Verification items for the finished model (mm, model axes). A direction names the side the tool comes from. Coordinates: 2 decimals unless noted, no trailing zeros. Order: outer loops, then holes, each group sorted by start corner. A loop starts at its lowest first (then second) coordinate and runs counter-clockwise, first axis right, second up. Notation, with made-up numbers: M 34,-21.5 L 38,-21.5 A31 ccw 38,4.5 Z; hole C 17,40.25 d6. An arc over 180 degrees is marked long. Return JSON: item names as keys, results as strings. Group by question number.
1. Material ranges on line 1 along Y through (x, z) = (-21.5, 0.9); line 2 along X through (y, z) = (18, 0.2); line 3 along Y through (x, z) = (0, 0.8), recorded low to high.
2. Section check B-B, the plane y = 15.5. Record the cut outline in (x, z), plus the area to 3 significant figures.
3. Section check D-D, the plane z = 1.25. Give the number of separate pieces and of enclosed holes in the cut face, plus the area to 3 significant figures.
4. Gauge pin test, flat ends, axial feed: pin 1 (12 mm diameter, centred on x = -15, y = 5, fed in from +Z); pin 2 (0.8 mm diameter, centred on y = -10.5, z = 0.5, fed in from +X). Record the tip position at first contact, or that the pin passes through.
5. Section check A-A, the plane x = -23.46. Record the cut outline in (y, z).
6. Set-up check for faces 4 (the cylindrical face through (-27.78, 10.25, 0.76)), 5 (the flat face through (2, -12, 1)), 6 (the cylindrical face through (2.179, 7.967, 0.76)): record each of +Z, -Z, +X, -X, +Y, -Y from which the full face is reachable in a straight line by a thin tool's end or side.
7. Section check C-C, the plane x = 5.5. Record the cut outline in (y, z), plus the area to 3 significant figures.
8. Mould release check, pull along X, two halves, no side actions. Record for faces 1 (the flat face through (2, 17, 1)), 2 (the flat face through (-31, 6, 1)), 3 (the flat face through (-4.49, 23, 1)): +X half, -X half, draft (parallel to the pull), parting line (faces both ways), or undercut.
Autodesk Inventor part; units mm, degrees
ref_plane "YZ Plane" through (0, 0, 0) normal (1, 0, 0) x (0, 1, 0)
ref_plane "XZ Plane" through (0, 0, 0) normal (0, 1, 0) x (-1, 0, 0)
ref_plane "XY Plane" through (0, 0, 0) normal (0, 0, 1) x (1, 0, 0)
sketch "スケッチ1" plane through (0, 0, 0) normal (0, 0, 1) x (1, 0, 0)
  circle A0 centre (0, 0) radius 6.05
  arc A1 (2, -7.7976) -> (2, 7.7976) centre (0, 0) ccw
  line L0 (-31, 0) -> (0, 0) construction
  line L1 (-24.51, 24.01) -> (-4.49, 24.01)
  line L2 (-4.49, 24.01) -> (-4.49, 21.99)
  line L3 (-4.49, 21.99) -> (-24.51, 21.99)
  line L4 (-24.51, 21.99) -> (-24.51, 24.01)
  line L5 (-24.51, 24.01) -> (-4.49, 21.99) construction
  line L6 (-4.49, 24.01) -> (-24.51, 21.99) construction
  line L7 (-24.5, 24) -> (-4.5, 24) construction
  line L8 (-4.5, 24) -> (-4.5, 22) construction
  line L9 (-4.5, 22) -> (-24.5, 22) construction
  line L10 (-24.5, 22) -> (-24.5, 24) construction
  line L11 (-24.5, 24) -> (-4.5, 22) construction
  line L12 (-4.5, 24) -> (-24.5, 22) construction
  line L13 (-24.51, 23) -> (-4.49, 23) construction
  arc A2 (-22.41, 24.01) -> (-24.51, 24.01) centre (-23.46, 24.01) ccw
  arc A3 (-24.51, 21.99) -> (-22.41, 21.99) centre (-23.46, 21.99) ccw
  line L14 (-14.5, 24) -> (-14.5, 21.99) construction
  arc A4 (-4.49, 24.01) -> (-6.59, 24.01) centre (-5.54, 24.01) ccw
  arc A5 (-6.59, 21.99) -> (-4.49, 21.99) centre (-5.54, 21.99) ccw
  line L15 (-28, 13.5) -> (-1, 13.5) construction
  line L16 (-1, 13.5) -> (-1, -13.5) construction
  line L17 (-1, -13.5) -> (-28, -13.5) construction
  line L18 (-28, -13.5) -> (-28, 13.5) construction
  line L19 (-28, 13.5) -> (-1, -13.5) construction
  line L20 (-1, 13.5) -> (-28, -13.5) construction
  line L21 (-14.5, 13.5) -> (-14.5, -13.5) construction
  line L22 (-24.51, -10.49) -> (-4.49, -10.49)
  line L23 (-4.49, -10.49) -> (-4.49, -12.51)
  line L24 (-4.49, -12.51) -> (-24.51, -12.51)
  line L25 (-24.51, -12.51) -> (-24.51, -10.49)
  line L26 (-24.51, -10.49) -> (-4.49, -12.51) construction
  line L27 (-4.49, -10.49) -> (-24.51, -12.51) construction
  line L28 (-24.5, -10.5) -> (-4.5, -10.5) construction
  line L29 (-4.5, -10.5) -> (-4.5, -12.5) construction
  line L30 (-4.5, -12.5) -> (-24.5, -12.5) construction
  line L31 (-24.5, -12.5) -> (-24.5, -10.5) construction
  line L32 (-24.5, -10.5) -> (-4.5, -12.5) construction
  line L33 (-4.5, -10.5) -> (-24.5, -12.5) construction
  line L34 (-24.51, -11.5) -> (-4.49, -11.5) construction
  arc A6 (-22.41, -10.49) -> (-24.51, -10.49) centre (-23.46, -10.49) ccw
  arc A7 (-24.51, -12.51) -> (-22.41, -12.51) centre (-23.46, -12.51) ccw
  line L35 (-14.5, -10.5) -> (-14.5, -12.51) construction
  arc A8 (-4.49, -10.49) -> (-6.59, -10.49) centre (-5.54, -10.49) ccw
  arc A9 (-6.59, -12.51) -> (-4.49, -12.51) centre (-5.54, -12.51) ccw
  line L36 (-31, 27) -> (-31, -16.5)
  line L37 (-31, -16.5) -> (2, -16.5)
  line L38 (2, -16.5) -> (2, -7.7976)
  line L39 (2, 7.7976) -> (2, 27)
  line L40 (2, 27) -> (-31, 27)
  arc A10 (-28, 10.5) -> (-25, 13.5) centre (-28, 13.5) ccw
  line L41 (-28, 10.5) -> (-28, 10.5)
  line L42 (-28, 10.5) -> (-28, -7.5)
  line L43 (-28, -7.5) -> (-8.05, -7.5)
  line L44 (-8.05, -7.5) -> (-8.05, 0)
  line L45 (-25, 13.5) -> (-25, 19)
  line L46 (-25, 19) -> (-4, 19)
  arc A11 (-1, 7.9876) -> (-8.05, 0) centre (0, 0) ccw
  line L47 (-1, 9.5) -> (-1, 7.9876)
  circle A12 centre (-28, 13.5) radius 1.35
  arc A13 (0.35, 13.5) -> (-2.35, 13.5) centre (-1, 13.5) ccw
  arc A14 (-2.35, 12.5) -> (0.35, 12.5) centre (-1, 12.5) ccw
  arc A15 (-4, 12.5) -> (-1, 9.5) centre (-1, 12.5) ccw
  line L48 (0.35, 12.5) -> (0.35, 13.5)
  line L49 (-2.35, 13.5) -> (-2.35, 12.5)
  line L50 (-4, 19) -> (-4, 12.5)
  arc A16 (-2.35, -13.5) -> (0.35, -13.5) centre (-1, -13.5) ccw
  arc A17 (0.35, -12.5) -> (-2.35, -12.5) centre (-1, -12.5) ccw
  line L51 (0.35, -12.5) -> (0.35, -13.5)
  line L52 (-2.35, -13.5) -> (-2.35, -12.5)
  circle A18 centre (-28, -13.5) radius 1.35
  point P0 (-14.5, 23)
  point P1 (-14.5, 0)
  point P2 (-14.5, -11.5)
  point P3 (-14.5, 22.995)
  point P4 (-6.59, -10.49)
  point P5 (-6.59, -12.51)
  point P6 (-22.41, -12.51)
  point P7 (-6.59, 24.01)
  dimension "d96" = 12.1
  dimension "d215" = 20
  dimension "d216" = 2
  dimension "d217" = 0.01
  dimension "d219" = 0.01
  dimension "d220" = 1.05
  dimension "d222" = 27
  dimension "d223" = 27
  dimension "d226" = 20
  dimension "d227" = 2
  dimension "d228" = 0.01
  dimension "d229" = 0.01
  dimension "d230" = 1.05
  dimension "d231" = 32.5
  dimension "d238" = 3
  dimension "d240" = 3
  dimension "d241" = 3
  dimension "d242" = 4
  dimension "d243" = 3
  dimension "d244" = 2
  dimension "d245" = 3
  dimension "d246" = 3
  dimension "d247" = 3
  dimension "d248" = 3
  dimension "d251" = 2
  dimension "d252" = 3
  dimension "d255" = 1
  dimension "d257" = 2.7
  dimension "d259" = 2.7
  dimension "d260" = 1
  dimension "d262" = 3
extrude "押し出し1" add sketch "スケッチ1" along normal blind 1.5
fillet "フィレット1" radius 1 7 edges at (-1, 7.9876, 0.75) (-8.05, -7.5, 0.75) (-28, -7.5, 0.75) (-25, 19, 0.75) (-28, 10.5, 0.75) (-4, 19, 0.75) (-1, 9.5, 0.75)
fillet "フィレット2" radius 1 6 edges at (-31, 27, 0.75) (2, 27, 0.75) (-31, -16.5, 0.75) (2, -7.7976, 0.75) (2, -16.5, 0.75) (2, 7.7976, 0.75)
properties part number "Trunk_vertical_frame_06" material "アルミニウム 2014-T4"
Answers follow:
{
 "1": {"line 1": "-16.5 to -12.51, -10.49 to -7.5, 19 to 21.99, 24.01 to 27", "line 2": "-31 to -25, -4 to 2", "line 3": "-16.5 to -14.41, -11.59 to -6.05, 6.05 to 11.59, 14.41 to 27"},
 "2": {"outline": "M -31,0 L -25,0 L -25,1.5 L -31,1.5 Z; M -4,0 L 2,0 L 2,1.5 L -4,1.5 Z", "area": "18.0 mm^2"},
 "3": {"separate pieces": "1", "enclosed holes": "8", "area": "699 mm^2"},
 "4": {"pin 1": "through", "pin 2": "x = 2"},
 "5": {"outline": "M -16.5,0 L -13.56,0 L -13.56,1.5 L -16.5,1.5 Z; M -9.44,0 L -7.5,0 L -7.5,1.5 L -9.44,1.5 Z; M 19,0 L 20.94,0 L 20.94,1.5 L 19,1.5 Z; M 25.06,0 L 27,0 L 27,1.5 L 25.06,1.5 Z"},
 "6": {"face 4": "+Z, -Z", "face 5": "+Z, -Z, +X, -Y", "face 6": "+Z, -Z, +X, +Y"},
 "7": {"outline": "M -5.88,0 L -2.52,0 L -2.52,1.5 L -5.88,1.5 Z; M 2.52,0 L 5.88,0 L 5.88,1.5 L 2.52,1.5 Z", "area": "10.1 mm^2"},
 "8": {"face 1": "+X half", "face 2": "-X half", "face 3": "undercut"}
}
